from build123d import *

# Parameters (mm, degrees)
BOSS_EXTRUDE1_DEPTH = 8.5
SKETCH2_R           = 0.9
SKETCH2_R_2         = 1.4
CUT_EXTRUDE1_DEPTH  = 14.592277219
CUT_EXTRUDE2_DEPTH  = 14.592277219
CUT_EXTRUDE3_REACH  = 22.037
CUT_EXTRUDE4_REACH  = 22.037
FILLET1_R           = 1


with BuildPart() as part:
    # Sketch1 → Boss-Extrude1 (new, symmetric)
    with BuildSketch(Plane.XY):
        Polygon((-5, 0), (5, 0), (5.769932482, -0.5), (10.5, -0.5), (10.5, -1.5), (5.487, -1.5), (4.717067518, -1), (-4.717067518, -1), (-5.487, -1.5), (-10.5, -1.5), (-10.5, -0.5), (-5.769932482, -0.5), align=None)
    extrude(amount=BOSS_EXTRUDE1_DEPTH, both=True)

    # Sketch2 → Cut-Extrude1 (cut, through all)
    with BuildSketch(Plane(origin=(0, 0, 0), x_dir=(1, 0, 0), z_dir=(0, 1, 0))):
        with Locations(Location((-3.3, -6.8, 0), (0, 0, 270))):
            Circle(SKETCH2_R)
        with Locations(Location((3.3, -6.8, 0), (0, 0, 270))):
            Circle(SKETCH2_R)
        with Locations(Location((8, -4.5, 0), (0, 0, 270))):
            Circle(SKETCH2_R_2)
        with Locations(Location((-8, 4.5, 0), (0, 0, 270))):
            Circle(SKETCH2_R_2)
    extrude(amount=-CUT_EXTRUDE1_DEPTH, mode=Mode.SUBTRACT)

    # Sketch3 → Cut-Extrude2 (cut, through all)
    with BuildSketch(Plane(origin=(0, 0, 0), x_dir=(1, 0, 0), z_dir=(0, 1, 0))):
        Polygon((5, -8.5), (10.5, -7.530201606), (10.5, -8.5), align=None)
        Polygon((10.5, -1.38), (5, -0.410201606), (5, 8.5), (10.5, 8.5), align=None)
        Polygon((-10.5, 8.5), (-5, 8.5), (-10.5, 7.530201606), align=None)
        Polygon((-10.5, 1.38), (-5, 0.410201606), (-5, -8.5), (-10.5, -8.5), align=None)
    extrude(amount=-CUT_EXTRUDE2_DEPTH, mode=Mode.SUBTRACT)

    # Cut-Extrude3: up to this face of the body (flat: up to its plane)
    cut_extrude3_end = Plane(part.part.faces().sort_by_distance((-7.700021392, -0.971737286, -0.886288226))[0])
    # Sketch4 → Cut-Extrude3 (cut, up to the picked face)
    with BuildSketch(Plane.XY.offset(8.5), mode=Mode.PRIVATE) as cut_extrude3_sk1:
        Polygon((-5, -1.183738502), (-4.717067518, -1), (-5, -1), align=None)
    cut_extrude3_tool1 = split(extrude(cut_extrude3_sk1.sketch, amount=-CUT_EXTRUDE3_REACH, mode=Mode.PRIVATE), bisect_by=cut_extrude3_end, keep=Keep.BOTH, mode=Mode.PRIVATE)
    add(cut_extrude3_tool1.solids().sort_by(Axis((-4.905689, -1.061246, 8.5), (0, 0, -1)))[0], mode=Mode.SUBTRACT)

    # Cut-Extrude4: up to this face of the body (flat: up to its plane)
    cut_extrude4_end = Plane(part.part.faces().sort_by_distance((7.700021392, -0.971737286, 0.886288226))[0])
    # Sketch5 → Cut-Extrude4 (cut, up to the picked face)
    with BuildSketch(Plane(origin=(0, 0, -8.5), x_dir=(-1, 0, 0), z_dir=(0, 0, -1)), mode=Mode.PRIVATE) as cut_extrude4_sk1:
        Polygon((-5, -1.183738502), (-4.717067518, -1), (-5, -1), align=None)
    cut_extrude4_tool1 = split(extrude(cut_extrude4_sk1.sketch, amount=-CUT_EXTRUDE4_REACH, mode=Mode.PRIVATE), bisect_by=cut_extrude4_end, keep=Keep.BOTH, mode=Mode.PRIVATE)
    add(cut_extrude4_tool1.solids().sort_by(Axis((4.905689, -1.061246, -8.5), (0, 0, 1)))[0], mode=Mode.SUBTRACT)

    # Fillet1
    fillet1_edges = [part.edges().sort_by_distance(p)[0] for p in [
        (-10.5, -1, -1.38),
        (10.5, -1, 7.530201606),
        (10.5, -1, 1.38),
        (-10.5, -1, -7.530201606),
    ]]
    fillet(fillet1_edges, radius=FILLET1_R)


solid = part.part
Geometry check sheet. Reference: the model listing, model coordinates, mm. A direction names the side the tool comes from. Round coordinates to 2 decimals unless told otherwise and drop trailing zeros. Order: outer loops, then holes, each group sorted by start corner. A loop starts at its lowest first (then second) coordinate and runs counter-clockwise, first axis right, second up. Notation, with made-up numbers: M 57.5,-25.75 L 61.5,-25.75 A16 ccw 61.5,-16.75 Z; hole C 72.5,5 d10. An arc over 180 degrees is marked long. Answer in a Markdown table with one row per item.
(1) Tool access check on faces 1 (the face through (6, -1.5, 5)), 2 (the face through (-9.2, -0.5, -3.5)). Record the directions out of +Z, -Z, +X, -X, +Y, -Y that give a thin tool (end or side, any length) a straight path to the whole face; none if there is none.
Responses:
| item | result |
|---|---|
| face 1 | +Z, -Z, +X, -X, -Y |
| face 2 | +Z, -Z, -X, +Y |
(2) Sectioned sample at C-C, the plane z = -6.25. Record the cut outline in (x, y).
Responses:
| item | result |
|---|---|
| outline | M -10.5,-1.5 L -5.49,-1.5 L -4.72,-1 L 5,-1 L 5,0 L -5,0 L -5.77,-0.5 L -10.5,-0.5 Z |
(3) Scan lines: probe 1 along X at (y, z) = (-0.65, 6.8); probe 2 along X at (y, z) = (-0.2, 6.8); probe 3 along Y at (x, z) = (-2.5, -0.25). Record each from-to range of solid material in increasing order. Write a range as from..to.
Responses:
| item | result |
|---|---|
| probe 1 | x = -5..-4.2, -2.4..2.4, 4.2..10.49 |
| probe 2 | x = -5..-4.2, -2.4..2.4, 4.2..5.31 |
| probe 3 | y = -1..0 |
(4) Sectioned sample at B-B, the plane x = 3.3. Record the cut outline in (y, z).
Responses:
| item | result |
|---|---|
| outline | M -1,-8.5 L 0,-8.5 L 0,5.9 L -1,5.9 Z; M -1,7.7 L 0,7.7 L 0,8.5 L -1,8.5 Z |
(5) Go/stop test with flat-tipped pins: P1, Ø1.1, axis at x = -3.3, z = 6.8, coming from the -Y side; P2, Ø10, axis at x = -4, z = 1.5, coming from the +Y side; P3, Ø0.8, axis at y = -0.5, z = -2.5, coming from the +X side; P4, Ø3, axis at x = 3.3, z = 6.8, coming from the -Y side. Record where each tip stops, or that it passes through.
Responses:
| item | result |
|---|---|
| P1 | passes through |
| P2 | stops at y = 0 |
| P3 | stops at x = 5 |
| P4 | stops at y = -1.05 |
(6) Sectioned sample at D-D, the plane z = 5.5. Record the cut outline in (x, y), and give its area (3 significant figures).
Responses:
| item | result |
|---|---|
| outline | M -5,-1 L 4.72,-1 L 5.49,-1.5 L 7.02,-1.5 L 7.02,-0.5 L 5.77,-0.5 L 5,0 L -5,0 Z; M 8.98,-1.5 L 10.5,-1.5 L 10.5,-0.5 L 8.98,-0.5 Z |
| area | 13.7 mm² |
(7) Sectioned sample at A-A, the plane z = -4.5. Record the cut outline in (x, y), and give its area (3 significant figures).
Responses:
| item | result |
|---|---|
| outline | M -10.5,-1.5 L -9.4,-1.5 L -9.4,-0.5 L -10.5,-0.5 Z; M -6.6,-1.5 L -5.49,-1.5 L -4.72,-1 L 5,-1 L 5,0 L -5,0 L -5.77,-0.5 L -6.6,-0.5 Z |
| area | 12.8 mm² |
